Build history of the part. All positions in model axes, mm. A direction names the side the tool comes from. Round coordinates to 2 decimals unless told otherwise and drop trailing zeros. Write each loop counter-clockwise with the first axis right and the second up, starting at its lowest first coordinate (ties: lowest second). Pieces come first, ordered by that corner, then holes. Notation, with made-up numbers: (84, 77.25) -> (106, 77.25) arc R24 cw to (106, 88.25) -> close; hole circle Ø11 at (69.25, -36.5). An arc over 180 degrees is marked (long way). Answer in a Markdown table with one row per item.
```python
from build123d import *

# Parameters (mm, degrees)
SKETCH_1_R               = 27.5
EXTRUDE_1_DEPTH          = 3
SKETCH_2_R               = 15
EXTRUDE_2_DEPTH          = 5
CUT_EXTRUDE_1_REACH      = 41.211
SKETCH_4_R               = 1.6
PATTERN_CIRCULAR_1_COUNT = 6
SKETCH_5_R               = 8
CUT_EXTRUDE_2_DEPTH      = 5


with BuildPart() as part:
    # 草图1 → 凸台-拉伸1 (new body)
    with BuildSketch(Plane(origin=(0, 0, 0), x_dir=(1, 0, 0), z_dir=(0, 1, 0))):
        with Locations(Location((0, 0, 0), (0, 0, 270))):
            Circle(SKETCH_1_R)
    extrude(amount=EXTRUDE_1_DEPTH)

    # 草图2 → 凸台-拉伸2 (add)
    with BuildSketch(Plane(origin=(0, 3, 0), x_dir=(1, 0, 0), z_dir=(0, 1, 0))):
        with Locations(Location((0, 0, 0), (0, 0, 270))):
            Circle(SKETCH_2_R)
    extrude(amount=EXTRUDE_2_DEPTH)

    # 草图4 → 切除-拉伸1 (cut, up to next)
    with BuildSketch(Plane(origin=(0, 3, 0), x_dir=(1, 0, 0), z_dir=(0, 1, 0)), mode=Mode.PRIVATE) as cut_extrude_1_sk1:
        with Locations(Location((0, 24, 0), (0, 0, 270))):
            Circle(SKETCH_4_R)
    cut_extrude_1_tool1 = extrude(cut_extrude_1_sk1.sketch, amount=-CUT_EXTRUDE_1_REACH, mode=Mode.PRIVATE) & part.part
    cut_extrude_1 = cut_extrude_1_tool1.solids().sort_by_distance((0, 3, -24))[0]
    add(cut_extrude_1, mode=Mode.SUBTRACT)

    # 阵列(圆周)1: 切除-拉伸1 ×6 about axis
    pattern_circular_1_axis = Axis((0, 0, 0), (0, 1, 0))
    for i in range(1, PATTERN_CIRCULAR_1_COUNT):
        add(cut_extrude_1.rotate(pattern_circular_1_axis, i * 360 / PATTERN_CIRCULAR_1_COUNT), mode=Mode.SUBTRACT)

    # 草图5 → 切除-拉伸2 (cut)
    with BuildSketch(Plane(origin=(0, 8, 0), x_dir=(1, 0, 0), z_dir=(0, 1, 0))):
        with Locations(Location((0, 0, 0), (0, 0, 270))):
            Circle(SKETCH_5_R)
    extrude(amount=-CUT_EXTRUDE_2_DEPTH, mode=Mode.SUBTRACT)


solid = part.part
```
Q1. Saw through at D-D on y = 1. Write the cut outline in (x, z), plus the area to 3 significant figures.
A:
| item | result |
|---|---|
| outline | circle Ø55 at (0, 0); hole circle Ø3.2 at (-20.78, -12); hole circle Ø3.2 at (-20.78, 12); hole circle Ø3.2 at (0, -24); hole circle Ø3.2 at (0, 24); hole circle Ø3.2 at (20.78, -12); hole circle Ø3.2 at (20.78, 12) |
| area | 2,330 mm² |
Q2. Saw through at A-A on z = -24. Write the cut outline in (x, y).
A:
| item | result |
|---|---|
| outline | (-13.43, 0) -> (-1.6, 0) -> (-1.6, 3) -> (-13.43, 3) -> close; (1.6, 0) -> (13.43, 0) -> (13.43, 3) -> (1.6, 3) -> close |
Q3. Which spindle directions (+Z, -Z, +X, -X, +Y, -Y) get a long thin tool onto all of the face, cutting with end or side? Do faces 1 (the flat face through (-12, 3, 12)), 2 (the cylindrical face through (19.223, 1.521, 11.653)). Say none if no direction does.
A:
| item | result |
|---|---|
| face 1 | +Y |
| face 2 | +Y, -Y |
Q4. Wall check: line 1 (X direction, y = 0.65, z = 12); line 2 (X direction, y = 1, z = 12.5); line 3 (Y direction, x = 13.5, z = 16). Give the ranges that are in metal, low to high. Write a range as [from, to].
A:
| item | result |
|---|---|
| line 1 | [-24.74, -22.38], [-19.18, 19.18], [22.38, 24.74] |
| line 2 | [-24.49, -22.3], [-19.26, 19.26], [22.3, 24.49] |
| line 3 | [0, 3] |
Q5. Drop flat-ended pins along their axis: P1, Ø5, axis at x = 20.78, z = 12, coming from the -Y side; P2, Ø5, axis at x = 20.78, z = -12, coming from the +Y side; P3, Ø4, axis at y = 4, z = -1, coming from the -X side. Give the stop position or say it passes through.
A:
| item | result |
|---|---|
| P1 | y = 0 |
| P2 | y = 3 |
| P3 | x = -27.5 |
Q6. Two-plate mould, pull along X, no slides. Class faces 3 (the flat face through (-6, 8, 6)), 4 (the cylindrical face through (-7.81, 5.54, -1.73)), 5 (the cylindrical face through (0.66, 5.465, -14.985)): released by +X, released by -X, zero draft, split by the parting line, or undercut.
A:
| item | result |
|---|---|
| face 3 | zero draft |
| face 4 | undercut |
| face 5 | split by the parting line |
Q7. Saw through at B-B on x = 0. Write the cut outline in (y, z), plus the area to 3 significant figures.
A:
| item | result |
|---|---|
| outline | (0, -27.5) -> (3, -27.5) -> (3, -25.6) -> (0, -25.6) -> close; (0, -22.4) -> (3, -22.4) -> (3, -15) -> (8, -15) -> (8, -8) -> (3, -8) -> (3, 8) -> (8, 8) -> (8, 15) -> (3, 15) -> (3, 22.4) -> (0, 22.4) -> close; (0, 25.6) -> (3, 25.6) -> (3, 27.5) -> (0, 27.5) -> close |
| area | 216 mm² |
Q8. Saw through at C-C on z = 12. Write the cut outline in (x, y), plus the area to 3 significant figures.
A:
| item | result |
|---|---|
| outline | (-24.74, 0) -> (-22.38, 0) -> (-22.38, 3) -> (-24.74, 3) -> close; (-19.18, 0) -> (19.18, 0) -> (19.18, 3) -> (9, 3) -> (9, 8) -> (-9, 8) -> (-9, 3) -> (-19.18, 3) -> close; (22.38, 0) -> (24.74, 0) -> (24.74, 3) -> (22.38, 3) -> close |
| area | 219 mm² |
